```python
from build123d import *

# Parameters (mm, degrees)
BASE_30_MM_DEPTH = 25
BASE_32_MM_DEPTH = 20
ESQUISSE5_R      = 2
VIDE_VIS_DEPTH   = 16.696819514


with BuildPart() as part:
    # Esquisse1 → BASE - 30 mm (new body)
    with BuildSketch(Plane.XY):
        with BuildLine():
            Line((30, 0), (15, 0))
            ThreePointArc((15, 0), (0, -15), (-15, 0))
            Line((-15, 0), (-30, 0))
            Line((-30, 0), (-30, -16.696819514))
            Line((-30, -16.696819514), (30, -16.696819514))
            Line((30, -16.696819514), (30, 0))
        make_face()
    extrude(amount=BASE_30_MM_DEPTH)

    # Esquisse4 → BASE - 32 mm (add)
    with BuildSketch(Plane.XY):
        with BuildLine():
            Line((20, 0), (30, 0))
            Line((30, 0), (30, -16.696819514))
            Line((30, -16.696819514), (-30, -16.696819514))
            Line((-30, -16.696819514), (-30, 0))
            Line((-30, 0), (-20, 0))
            Line((-20, 0), (-16, 0))
            ThreePointArc((-16, 0), (0, -16), (16, 0))
            Line((16, 0), (20, 0))
        make_face()
    extrude(amount=-BASE_32_MM_DEPTH)

    # Esquisse5 → VIDE VIS (cut)
    with BuildSketch(Plane.XZ.offset(16.696819514)):
        with Locations(Location((-23, -10, 0), (0, 0, 270))):
            Circle(ESQUISSE5_R)
        with Locations(Location((-22.5, 12.5, 0), (0, 0, 270))):
            Circle(ESQUISSE5_R)
        with Locations(Location((22.5, 12.5, 0), (0, 0, 270))):
            Circle(ESQUISSE5_R)
        with Locations(Location((23, -10, 0), (0, 0, 270))):
            Circle(ESQUISSE5_R)
    extrude(amount=-VIDE_VIS_DEPTH, mode=Mode.SUBTRACT)


solid = part.part
```
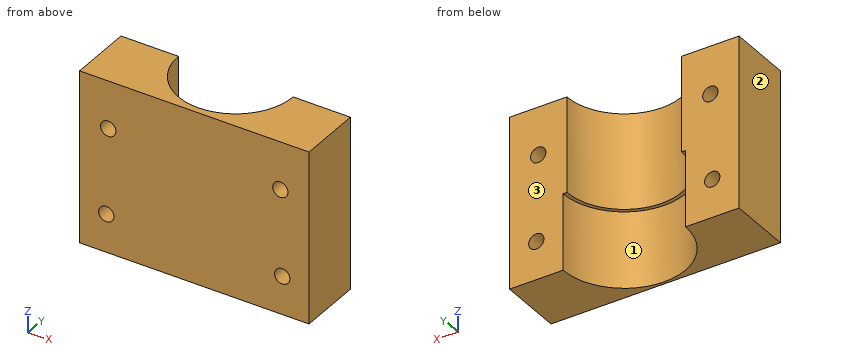
Input: part model. Units: mm. Frame: model coordinates. Face numbers are marked on the shaded views. Coordinates: 2 decimals unless noted, no trailing zeros. Loops run counter-clockwise (first coordinate to the right, second up) from the corner with the lowest first, then second, coordinate; pieces in that order, holes last. Notation, with made-up numbers: M -19,85.25 L 15,85.25 A9 cw 15,89.25 Z; hole C -29,53 d10. An arc over 180 degrees is marked long. Answer in a Markdown table with one row per item.
1. Section A-A, the plane z = -10. Output: boundary loops of the cut face in (x, y).
Response:
| item | result |
|---|---|
| outline | M -30,-16.7 L -25,-16.7 L -25,0 L -30,0 Z; M -21,-16.7 L 21,-16.7 L 21,0 L 16,0 A16 cw -16,0 L -21,0 Z; M 25,-16.7 L 30,-16.7 L 30,0 L 25,0 Z |
2. Section D-D, the plane y = -11. Output: boundary loops of the cut face in (x, z), then the cut area to 3 significant figures.
Response:
| item | result |
|---|---|
| outline | M -30,-20 L -11.62,-20 L -11.62,0 L -10.2,0 L -10.2,25 L -30,25 Z; M 10.2,0 L 11.62,0 L 11.62,-20 L 30,-20 L 30,25 L 10.2,25 Z; hole C -23,-10 d4; hole C -22.5,12.5 d4; hole C 22.5,12.5 d4; hole C 23,-10 d4 |
| area | 1,680 mm2 |
3. Section C-C, the plane x = 12.5. Output: boundary loops of the cut face in (y, z).
Response:
| item | result |
|---|---|
| outline | M -16.7,-20 L -9.99,-20 L -9.99,0 L -8.29,0 L -8.29,25 L -16.7,25 Z |
4. Draft query along X for the marked faces 1, 2 and 3. Return one class per face: pulls with the +X half, pulls with the -X half, needs draft (parallel to the pull), parting line crosses it, or undercut.
Response:
| item | result |
|---|---|
| face 1 | undercut |
| face 2 | pulls with the -X half |
| face 3 | needs draft |
5. Material intervals for line 1 (X direction, y = -11.5, z = 12.5); line 2 (X direction, y = -5.5, z = -10); line 3 (X direction, y = -3.25, z = 0.5), sorted ascending.
Response:
| item | result |
|---|---|
| line 1 | x = -30 to -24.5, -20.5 to -9.63, 9.63 to 20.5, 24.5 to 30 |
| line 2 | x = -30 to -25, -21 to -15.02, 15.02 to 21, 25 to 30 |
| line 3 | x = -30 to -14.64, 14.64 to 30 |
6. Section B-B, the plane y = -1. Output: boundary loops of the cut face in (x, z), then the cut area to 3 significant figures.
Response:
| item | result |
|---|---|
| outline | M -30,-20 L -15.97,-20 L -15.97,0 L -14.97,0 L -14.97,25 L -30,25 Z; M 14.97,0 L 15.97,0 L 15.97,-20 L 30,-20 L 30,25 L 14.97,25 Z; hole C -23,-10 d4; hole C -22.5,12.5 d4; hole C 22.5,12.5 d4; hole C 23,-10 d4 |
| area | 1,260 mm2 |
7. First-contact query: pin 1 (5 mm diameter, centred on x = -23, z = -13.5, fed in from +Y). Flat tip, straight axial feed; report the tip coordinate or a pass-through.
Response:
| item | result |
|---|---|
| pin 1 | stops at y = 0 |
